Geometry check sheet. Reference: the model listing, model coordinates, mm. Face numbers are marked on the shaded views. Give positions to 0.01 mm unless a question says otherwise; leave off trailing zeros. Loops run counter-clockwise (first coordinate to the right, second up) from the corner with the lowest first, then second, coordinate; pieces in that order, holes last. Notation, with made-up numbers: (38.25, 12.5) -> (96.25, 12.5) arc R18 cw to (96.25, 19.5) -> close; hole circle Ø10 at (35.25, -16.75). An arc over 180 degrees is marked (long way). Answer as a JSON object with one key per item and string values.
from build123d import *

# Parameters (mm, degrees)
F1_DEPTH = 52


with BuildPart() as f1:
    # F0 (on Front) → F1 (new body)
    with BuildSketch(Plane.XZ):
        with BuildLine():
            Line((-37.073477, 14.565424), (-39.125901, 9.761879))
            ThreePointArc((-39.125901, 9.761879), (-39.083382, 9.28995), (-38.666112, 9.065424))
            Line((-38.666112, 9.065424), (-17.966112, 9.065424))
            Line((-17.966112, 9.065424), (-17.966112, 10.765424))
            Line((-17.966112, 10.765424), (1.119158, 10.765424))
            Line((1.119158, 10.765424), (1.119158, 9.065424))
            Line((1.119158, 9.065424), (21.819158, 9.065424))
            ThreePointArc((21.819158, 9.065424), (22.236428, 9.28995), (22.278947, 9.761879))
            Line((22.278947, 9.761879), (20.226523, 14.565424))
            Line((20.226523, 14.565424), (22.278947, 19.677687))
            Line((22.278947, 19.677687), (22.278947, 21.677687))
            Line((22.278947, 21.677687), (-39.125901, 21.677687))
            Line((-39.125901, 21.677687), (-39.125901, 19.677687))
            Line((-39.125901, 19.677687), (-37.073477, 14.565424))
        make_face()
    extrude(amount=F1_DEPTH)


solid = f1.part
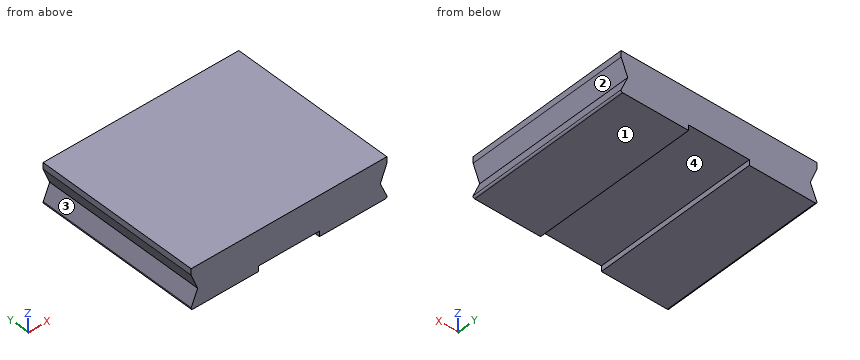
1) Section check C-C on z = 13.5. Record the cut outline in (x, y).
Geometry check:
{"outline": "(-37.53, -52) -> (20.68, -52) -> (20.68, 0) -> (-37.53, 0) -> close"}
2) Section check A-A on y = -27. Record the cut outline in (x, z), plus the area to 3 significant figures.
Geometry check:
{"outline": "(-39.13, 9.76) arc R0.5 ccw to (-38.67, 9.07) -> (-17.97, 9.07) -> (-17.97, 10.77) -> (1.12, 10.77) -> (1.12, 9.07) -> (21.82, 9.07) arc R0.5 ccw to (22.28, 9.76) -> (20.23, 14.57) -> (22.28, 19.68) -> (22.28, 21.68) -> (-39.13, 21.68) -> (-39.13, 19.68) -> (-37.07, 14.57) -> close", "area": "722 mm2"}
3) Material ranges on line 1 along X through (y, z) = (-39.5, 20.5); line 2 along Z through (x, y) = (-14, -3.5); line 3 along X through (y, z) = (-30.5, 10), recorded low to high. Write a range as from..to.
Geometry check:
{"line 1": "x = -39.13..22.28", "line 2": "z = 10.77..21.68", "line 3": "x = -39.02..-17.97, 1.12..22.18"}
4) Draft check along X on the marked faces 1, 2, 3 and 4. Enter one of: pulls with the +X half, pulls with the -X half, needs draft (parallel to the pull), parting line crosses it, or undercut.
Geometry check:
{"face 1": "needs draft", "face 2": "pulls with the +X half", "face 3": "pulls with the -X half", "face 4": "undercut"}
5) Depth check by flat-ended pin: P1, Ø2, axis at y = -32.5, z = 21, coming from the -X side; P2, Ø9.5, axis at x = -8.5, y = -21, coming from the -Z side; P3, Ø0.5, axis at y = -15.5, z = 10, coming from the +X side. Enter the tip coordinate at first touch or a pass-through.
Geometry check:
{"P1": "stops at x = -39.13", "P2": "stops at z = 10.77", "P3": "stops at x = 22.28"}
6) Section check B-B on x = -12.5. Record the cut outline in (y, z).
Geometry check:
{"outline": "(-52, 10.77) -> (0, 10.77) -> (0, 21.68) -> (-52, 21.68) -> close"}
